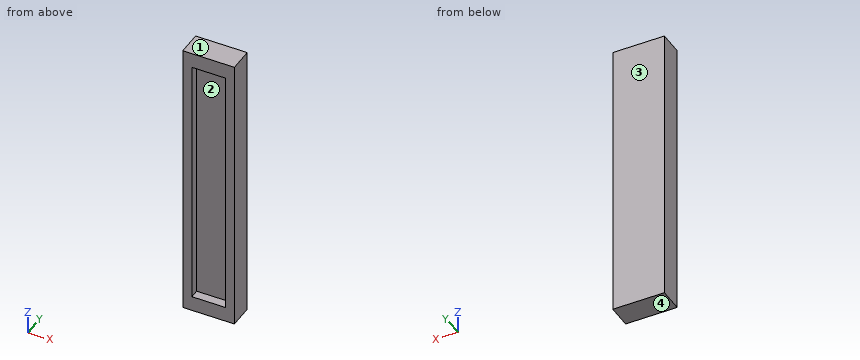
```python
from build123d import *

# Parameters (mm, degrees)
BOX009_W               = 84
BOX009_H               = 11
BOX009_DEPTH           = 5
BOX008_W               = 94
BOX008_H               = 17
BOX008_DEPTH           = 8
CUT009_PITCH_ANGLE     = 90
CUT009_PLACEMENT_ANGLE = 90


with BuildPart() as obj1:
    # Box009 → Box009 (new body)
    with BuildSketch(Plane.XY.offset(-2)):
        with Locations((42, 5.5)):
            Rectangle(BOX009_W, BOX009_H)
    extrude(amount=BOX009_DEPTH)


with BuildPart() as slidingmodule:
    # Box008 → Box008 (new body)
    with BuildSketch(Plane(origin=(-5, -3, 0), x_dir=(1, 0, 0), z_dir=(0, 0, 1))):
        with Locations((47, 8.5)):
            Rectangle(BOX008_W, BOX008_H)
    extrude(amount=BOX008_DEPTH)

    # Cut009: cut obj1
    add(obj1.part, mode=Mode.SUBTRACT)


with BuildPart() as slidingmodule_1:
    # Cut009 pitch: moved
    add(slidingmodule.part.rotate(Axis((0, 0, 0), (0, 1, 0)), CUT009_PITCH_ANGLE))


with BuildPart() as slidingmodule_2:
    # Cut009 placement: moved
    add(slidingmodule_1.part.moved(Location((26.65, 47.3, 41))).rotate(Axis((26.65, 47.3, 41), (0, 0, 1)), CUT009_PLACEMENT_ANGLE))


solid = slidingmodule_2.part
```
Verification items for the finished model (mm, model axes). Face numbers are marked on the shaded views. Round coordinates to 2 decimals unless told otherwise and drop trailing zeros. Order: outer loops, then holes, each group sorted by start corner. A loop starts at its lowest first (then second) coordinate and runs counter-clockwise, first axis right, second up. Notation, with made-up numbers: (13.25, 75.5) - (24.25, 75.5) arc R19 ccw to (24.25, 99.5) - close; hole circle Ø2 at (-35.75, 7.25). An arc over 180 degrees is marked (long way). Use CSV: the item, a comma, the result in double quotes. Start each with the question number.
1) Go/stop test with a flat-tipped pin: P1, Ø3, axis at x = 25, z = 20, coming from the -Y side. Record where the tip stops, or that it passes through.
2) Mould release check, pull along Z, two halves, no side actions. Record for the marked faces 1, 2, 3 and 4: +Z half, -Z half, draft (parallel to the pull), parting line (faces both ways), or undercut.
3) Section check B-B, the plane z = -19. Record the cut outline in (x, y).
4) Thickness scan on L1, parallel to X at y = 49.75, z = 7; L2, parallel to Z at x = 20.25, y = 49.5; L3, parallel to Y at x = 26.5, z = 24. Record the ranges inside material, lowest first.
5) Section check A-A, the plane x = 16.5. Record the cut outline in (y, z), plus the area to 3 significant figures.
Answers:
1,P1,"stops at y = 50.3"
2,face 1,"+Z half"
2,face 2,"undercut"
2,face 3,"draft"
2,face 4,"-Z half"
3,outline,"(12.65, 47.3) - (15.65, 47.3) - (15.65, 50.3) - (26.65, 50.3) - (26.65, 47.3) - (29.65, 47.3) - (29.65, 55.3) - (12.65, 55.3) - close"
4,L1,"x = 12.65 to 15.65, 26.65 to 29.65"
4,L2,"z = -48 to -43, 41 to 46"
4,L3,"y = 50.3 to 55.3"
5,outline,"(47.3, -48) - (55.3, -48) - (55.3, 46) - (47.3, 46) - (47.3, 41) - (50.3, 41) - (50.3, -43) - (47.3, -43) - close"
5,area,"500 mm²"
